from build123d import *

# Parameters (mm, degrees)
F1_DEPTH = 6.35
F2_R     = 9.525


with BuildPart() as f1:
    # F0 (on Front) → F1 (new body)
    with BuildSketch(Plane.XZ):
        with BuildLine():
            Line((25.583847, -6.35), (38.1, -6.35))
            Line((38.1, -6.35), (38.1, 6.35))
            Line((38.1, 6.35), (-38.1, 6.35))
            Line((-38.1, 6.35), (-38.1, -6.35))
            Line((-38.1, -6.35), (-29.139847, -6.35))
            ThreePointArc((-29.139847, -6.35), (-26.416, -0.508), (-23.692153, -6.35))
            Line((-23.692153, -6.35), (20.136153, -6.35))
            ThreePointArc((20.136153, -6.35), (22.86, -0.508), (25.583847, -6.35))
        make_face()
    extrude(amount=F1_DEPTH)

    # F2
    f2_edges = [f1.edges().sort_by_distance(p)[0] for p in [
        (-38.1, -3.175, 6.35),
        (38.1, -3.175, 6.35),
    ]]
    fillet(f2_edges, radius=F2_R)


solid = f1.part
Here's how the part is built. I have some questions about the finished solid (model axes, mm). Round coordinates to 2 decimals unless told otherwise and drop trailing zeros. Loops run counter-clockwise (first coordinate to the right, second up) from the corner with the lowest first, then second, coordinate; pieces in that order, holes last. Notation, with made-up numbers: (-26, 9.5) - (2, 9.5) arc R4 cw to (2, 15.5) - close; hole circle Ø8 at (3, 52.5). An arc over 180 degrees is marked (long way). One line per question, with ' | ' between items. Start each with the question number.
Q1. Please list where these lines run through material, in increasing order: line 1 (X direction, y = -2.5, z = -3.75); line 2 (X direction, y = -1.5, z = -5.25); line 3 (Z direction, x = 22.86, y = -2.25). Write a range as [from, to].
Q2. We'd pull the mould along X, two halves only. Please class faces 1 (the flat face through (-38.1, -3, -5)), 2 (the flat face through (32, -3, -6.35)), 3 (the cylindrical face through (22.75, -3.13, -0.51)), 4 (the flat face through (38.1, -3, -5)): +X half, -X half, draft (parallel to the pull), parting line (faces both ways), or undercut.
Q3. I want a section at A-A (y = -2.5). Write out the boundary of the cut face in (x, z) (3 decimals).
Q4. I want a section at C-C (z = 5.5). Write out the boundary of the cut face in (x, y), then the cut area to 3 significant figures.
Q5. I want a section at B-B (x = 22.86). Write out the boundary of the cut face in (y, z), then the cut area to 3 significant figures.
Response values:
1) line 1: x = [-38.1, -29.96], [-22.87, 19.32], [26.4, 38.1] | line 2: x = [-38.1, -29.77], [-23.06, 19.51], [26.21, 38.1] | line 3: z = [-0.51, 6.35]
2) face 1: -X half | face 2: draft | face 3: undercut | face 4: +X half
3) outline: (-38.1, -6.35) - (-29.14, -6.35) arc R3.556 cw (long way) to (-23.692, -6.35) - (20.136, -6.35) arc R3.556 cw (long way) to (25.584, -6.35) - (38.1, -6.35) - (38.1, -3.175) arc R9.525 ccw to (28.575, 6.35) - (-28.575, 6.35) arc R9.525 ccw to (-38.1, -3.175) - close
4) outline: (-32.51, -6.35) - (32.51, -6.35) - (32.51, 0) - (-32.51, 0) - close | area: 413 mm²
5) outline: (-6.35, -0.51) - (0, -0.51) - (0, 6.35) - (-6.35, 6.35) - close | area: 43.5 mm²
